The listing builds one solid part. Answer for the finished solid, in the listing's coordinates (mm). A direction names the side the tool comes from. Give positions to 0.01 mm unless a question says otherwise; leave off trailing zeros. Order: outer loops, then holes, each group sorted by start corner. A loop starts at its lowest first (then second) coordinate and runs counter-clockwise, first axis right, second up.
```python
from build123d import *

# Parameters (mm, degrees)
BOSS_EXTRUDE1_DEPTH   = 75
BOSS_EXTRUDE1_2_DEPTH = 75
BOSS_EXTRUDE2_DEPTH   = 45
SKETCH1_5_R           = 7.5
BOSS_EXTRUDE3_DEPTH   = 15
SKETCH2_R             = 6
CUT_EXTRUDE1_DEPTH    = 127.416968798


with BuildPart() as part:
    # Sketch1 → Boss-Extrude1 (new body)
    with BuildSketch(Plane(origin=(0, 0, 0), x_dir=(1, 0, 0), z_dir=(0, 1, 0))):
        with BuildLine():
            Line((24.366985862, 17.5), (-24.366985862, 17.5))
            ThreePointArc((-24.366985862, 17.5), (-27.171188586, 12.717173855), (-29.047375097, 7.5))
            Line((-29.047375097, 7.5), (29.047375097, 7.5))
            ThreePointArc((29.047375097, 7.5), (27.171188586, 12.717173855), (24.366985862, 17.5))
        make_face()
    extrude(amount=BOSS_EXTRUDE1_DEPTH)



with BuildPart() as body_2:
    # Sketch1 → Boss-Extrude1 2 (new body)
    with BuildSketch(Plane(origin=(0, 0, 0), x_dir=(1, 0, 0), z_dir=(0, 1, 0))):
        with BuildLine():
            ThreePointArc((-29.047375097, -7.5), (-27.171188586, -12.717173855), (-24.366985862, -17.5))
            Line((-24.366985862, -17.5), (24.366985862, -17.5))
            ThreePointArc((24.366985862, -17.5), (27.171188586, -12.717173855), (29.047375097, -7.5))
            Line((29.047375097, -7.5), (-29.047375097, -7.5))
        make_face()
    extrude(amount=BOSS_EXTRUDE1_2_DEPTH)


with BuildPart() as part_1:
    add(part.part)

    add(body_2.part)  # Boss-Extrude2 merges body 2
    # Sketch1_4 → Boss-Extrude2 (add)
    with BuildSketch(Plane(origin=(0, 0, 0), x_dir=(1, 0, 0), z_dir=(0, 1, 0))):
        with BuildLine():
            ThreePointArc((-24.366985862, -17.5), (-16.306579488, -25.18125226), (-6, -29.393876913))
            ThreePointArc((-6, -29.393876913), (0, -30), (6, -29.393876913))
            ThreePointArc((6, -29.393876913), (16.306579488, -25.18125226), (24.366985862, -17.5))
            Line((24.366985862, -17.5), (-24.366985862, -17.5))
        make_face()
        with BuildLine():
            ThreePointArc((-6, 29.393876913), (-16.306579488, 25.18125226), (-24.366985862, 17.5))
            Line((-24.366985862, 17.5), (24.366985862, 17.5))
            ThreePointArc((24.366985862, 17.5), (16.306579488, 25.18125226), (6, 29.393876913))
            ThreePointArc((6, 29.393876913), (0, 30), (-6, 29.393876913))
        make_face()
    extrude(amount=BOSS_EXTRUDE2_DEPTH)

    # Sketch1_5 → Boss-Extrude3 (add)
    with BuildSketch(Plane(origin=(0, 0, 0), x_dir=(1, 0, 0), z_dir=(0, 1, 0))):
        with BuildLine():
            ThreePointArc((-29.047375097, 7.5), (-27.171188586, 12.717173855), (-24.366985862, 17.5))
            ThreePointArc((-24.366985862, 17.5), (-16.306579488, 25.18125226), (-6, 29.393876913))
            Line((-6, 29.393876913), (-78, 14.696938457))
            ThreePointArc((-78, 14.696938457), (-90, 0), (-78, -14.696938457))
            Line((-78, -14.696938457), (-6, -29.393876913))
            ThreePointArc((-6, -29.393876913), (-16.306579488, -25.18125226), (-24.366985862, -17.5))
            ThreePointArc((-24.366985862, -17.5), (-27.171188586, -12.717173855), (-29.047375097, -7.5))
            Line((-29.047375097, -7.5), (29.047375097, -7.5))
            ThreePointArc((29.047375097, -7.5), (27.171188586, -12.717173855), (24.366985862, -17.5))
            ThreePointArc((24.366985862, -17.5), (16.306579488, -25.18125226), (6, -29.393876913))
            Line((6, -29.393876913), (78, -14.696938457))
            ThreePointArc((78, -14.696938457), (90, 0), (78, 14.696938457))
            Line((78, 14.696938457), (6, 29.393876913))
            ThreePointArc((6, 29.393876913), (16.306579488, 25.18125226), (24.366985862, 17.5))
            ThreePointArc((24.366985862, 17.5), (27.171188586, 12.717173855), (29.047375097, 7.5))
            Line((29.047375097, 7.5), (-29.047375097, 7.5))
        make_face()
        with Locations(Location((-75, 0, 0), (0, 0, 270))):
            Circle(SKETCH1_5_R, mode=Mode.SUBTRACT)
        with Locations(Location((75, 0, 0), (0, 0, 270))):
            Circle(SKETCH1_5_R, mode=Mode.SUBTRACT)
    extrude(amount=BOSS_EXTRUDE3_DEPTH)

    # Sketch2 → Cut-Extrude1 (cut, through all)
    with BuildSketch(Plane.XY.offset(17.5)):
        with Locations((0, 60)):
            Circle(SKETCH2_R)
    extrude(amount=-CUT_EXTRUDE1_DEPTH, mode=Mode.SUBTRACT)


solid = part_1.part
```
1) Find section A-A (y = 37). Write down the section's boundary in (x, z), then the cut area to 3 significant figures.
Geometry says:
outline: (-29.05, -7.5) arc R30 ccw to (29.05, -7.5) - close; (-29.05, 7.5) - (29.05, 7.5) arc R30 ccw to start
area: 1,940 mm2
2) Given P1, Ø15.5, axis at x = 0, y = 60, coming from the -Z side; P2, Ø4, axis at x = -2.5, z = -23, coming from the +Y side; P3, Ø12, axis at x = 29, y = 28.5, coming from the +Z side, each flat-ended and moving along its own axis, determine where each tip first touches the part or whether it passes through.
Geometry says:
P1: stops at z = -17.5
P2: stops at y = 45
P3: stops at z = 19.26
3) For a pull along X with two mould halves and no side action, classify faces 5 (the cylindrical face through (90, 7, 0)), 6 (the flat face through (-41.496, 7.395, -22.148)), 7 (the flat face through (0, 45, 7.5)), 8 (the cylindrical face through (-4.42, 64.06, -12.43)) as +X half, -X half, draft (parallel to the pull), parting line (faces both ways), or undercut.
Geometry says:
face 5: +X half
face 6: -X half
face 7: draft
face 8: undercut
4) Find section B-B (z = 0). Write down the section's boundary in (x, y).
Geometry says:
outline: (-90, 0) - (-82.5, 0) - (-82.5, 15) - (-90, 15) - close; (-67.5, 0) - (67.5, 0) - (67.5, 15) - (-67.5, 15) - close; (82.5, 0) - (90, 0) - (90, 15) - (82.5, 15) - close
5) Straight lines are drawn through the part: probe 1 along Y at (x, z) = (0, 13.75); probe 2 along Z at (x, y) = (-15.5, 66.5); probe 3 along Y at (x, z) = (-61, -11). For each, find the intervals that lie inside material, in ascending order.
Geometry says:
probe 1: y = 0 to 54, 66 to 75
probe 2: z = -17.5 to -7.5, 7.5 to 17.5
probe 3: y = 0 to 15
6) Find section C-C (y = 60). Write down the section's boundary in (x, z), then the cut area to 3 significant figures.
Geometry says:
outline: (-29.05, -7.5) arc R30 ccw to (-24.37, -17.5) - (-6, -17.5) - (-6, -7.5) - close; (-29.05, 7.5) - (-6, 7.5) - (-6, 17.5) - (-24.37, 17.5) arc R30 ccw to start; (6, -17.5) - (24.37, -17.5) arc R30 ccw to (29.05, -7.5) - (6, -7.5) - close; (6, 7.5) - (29.05, 7.5) arc R30 ccw to (24.37, 17.5) - (6, 17.5) - close
area: 843 mm2
7) Find section D-D (x = 0). Write down the section's boundary in (y, z), then the cut area to 3 significant figures.
Geometry says:
outline: (0, -30) - (45, -30) - (45, -17.5) - (54, -17.5) - (54, -7.5) - (15, -7.5) - (15, 7.5) - (54, 7.5) - (54, 17.5) - (45, 17.5) - (45, 30) - (0, 30) - close; (66, -17.5) - (75, -17.5) - (75, -7.5) - (66, -7.5) - close; (66, 7.5) - (75, 7.5) - (75, 17.5) - (66, 17.5) - close
area: 2,610 mm2
8) A tool of negligible diameter and unlimited length cuts with its end or side. For faces 1 (the flat face through (0, 45, 22)), 2 (the flat face through (0, 45, -7.5)), 3 (the flat face through (6, 56, -17.5)), 4 (the flat face through (-1, 15, 0)), from which of +Z, -Z, +X, -X, +Y, -Y can it reach the whole face along a straight path? Write none if from no direction.
Geometry says:
face 1: +Z, +X, -X, +Y
face 2: +X, -X, +Y
face 3: -Z, +X, -X, +Y
face 4: +Y
